from build123d import *

# Parameters (mm, degrees)
SKETCH1_W           = 40
SKETCH1_H           = 250
BOSS_EXTRUDE1_DEPTH = 6
CUT_EXTRUDE1_DEPTH  = 6


with BuildPart() as part:
    # Sketch1 → Boss-Extrude1 (new body)
    with BuildSketch(Plane.XY):
        Rectangle(SKETCH1_W, SKETCH1_H)
    extrude(amount=BOSS_EXTRUDE1_DEPTH)

    # Sketch2 → Cut-Extrude1 (cut)
    with BuildSketch(Plane.XY.offset(6)):
        with BuildLine():
            Line((-3.25, 125), (3.25, 125))
            Line((3.25, 125), (3.25, 55))
            ThreePointArc((3.25, 55), (0, 51.75), (-3.25, 55))
            Line((-3.25, 55), (-3.25, 125))
        make_face()
    extrude(amount=-CUT_EXTRUDE1_DEPTH, mode=Mode.SUBTRACT)


solid = part.part
Work out the finished part from the listing and answer in its coordinate system (mm). A direction names the side the tool comes from. Coordinates: 2 decimals unless noted, no trailing zeros. Write each loop counter-clockwise with the first axis right and the second up, starting at its lowest first coordinate (ties: lowest second). Pieces come first, ordered by that corner, then holes. Notation, with made-up numbers: (-6.5, 27.25) - (51.5, 27.25) arc R15 ccw to (51.5, 33.25) - close; hole circle Ø6 at (-7.5, 78). An arc over 180 degrees is marked (long way). One line per question, with ' | ' between items.
1) Find section C-C, the plane x = 0. Determine the outline of the cut face in (y, z), and give its area (3 significant figures).
Checks:
outline: (-125, 0) - (51.75, 0) - (51.75, 6) - (-125, 6) - close | area: 1,060 mm2
2) Find section B-B, the plane z = 0.9. Determine the outline of the cut face in (x, y).
Checks:
outline: (-20, -125) - (20, -125) - (20, 125) - (3.25, 125) - (3.25, 55) arc R3.25 cw to (-3.25, 55) - (-3.25, 125) - (-20, 125) - close
3) Find section A-A, the plane y = 99. Determine the outline of the cut face in (x, z).
Checks:
outline: (-20, 0) - (-3.25, 0) - (-3.25, 6) - (-20, 6) - close; (3.25, 0) - (20, 0) - (20, 6) - (3.25, 6) - close
4) Consider probe 1 along X at (y, z) = (82.5, 4.25); probe 2 along Y at (x, z) = (-1.5, 3.2). Determine where each line is inside the solid, lowest interval first. Write a range as [from, to].
Checks:
probe 1: [-20, -3.25], [3.25, 20] | probe 2: [-125, 52.12]
5) For faces 4 (the face through (3.25, 90, 3)), 5 (the face through (12, 125, 3)), determine the directions among +Z, -Z, +X, -X, +Y, -Y from which every point of the face is accessible in a straight line to the end or side of a thin tool.
Checks:
face 4: +Z, -Z, +Y | face 5: +Z, -Z, +X, -X, +Y
6) The mould has two halves that part along X. Classify faces 1 (the face through (-20, -2, 3)), 2 (the face through (-3.25, 90, 3)), 3 (the face through (0, 2, 0)): +X half, -X half, draft (parallel to the pull), parting line (faces both ways), or undercut.
Checks:
face 1: -X half | face 2: undercut | face 3: draft
